Could you check a few things on this drawing? It's one solid part, dimensions in mm from its lowest x, y, z. Give positions to 0.01 mm unless a question says otherwise; leave off trailing zeros. Order: outer loops, then holes, each group sorted by start corner. A loop starts at its lowest first (then second) coordinate and runs counter-clockwise, first axis right, second up. Notation, with made-up numbers: (-19, 0) -> (9, 0) arc R19 cw to (9, 24) -> close; hole circle Ø11 at (67, 85.25). An arc over 180 degrees is marked (long way). Use one line per item in the form item = value. Start each with the question number.
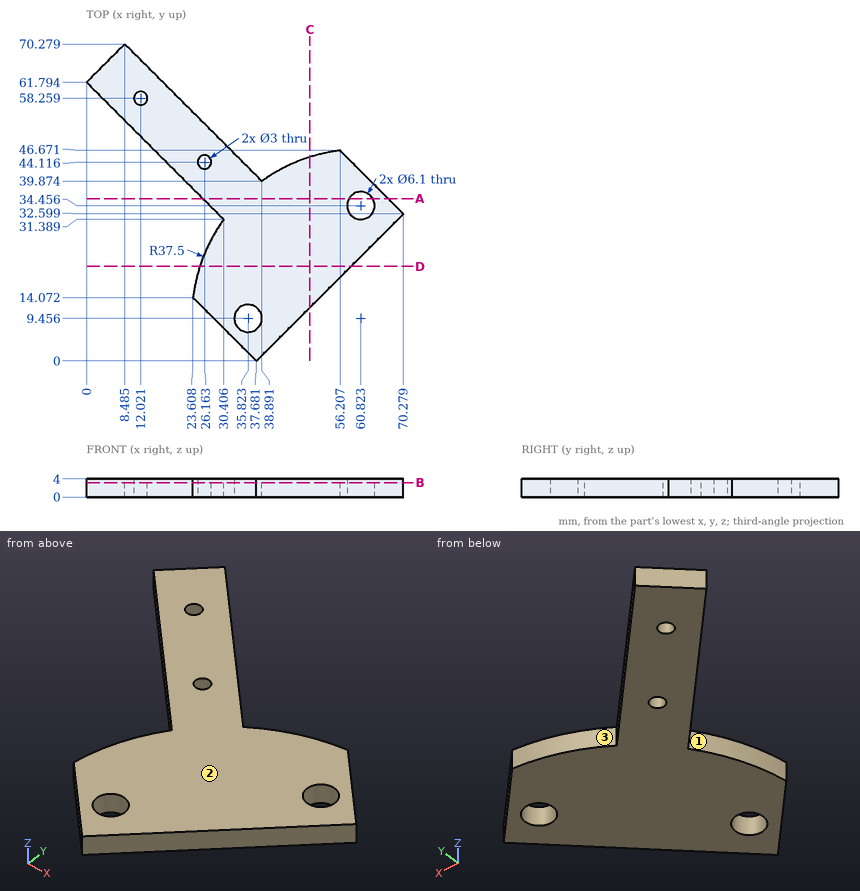
(1) I'm going to push flat-ended pins straight in: pin 1 Ø2.5 at (x, y) = (26.16, 44.12) entering from +Z; pin 2 Ø1 at (x, z) = (25, 3.5) entering from -Y; pin 3 Ø2 at (x, z) = (16.5, 3) entering from -Y (1 decimal). Where does each tip first touch, or does it pass through?
(2) Please list where these lines run through material, in increasing order: probe 1 along Y at (x, z) = (35.5, 3.35) (1 decimal); probe 2 along X at (y, z) = (40, 1.7) (1 decimal); probe 3 along X at (y, z) = (34, 1.95) (1 decimal).
(3) Imagine slicing it at D-D (y = 21). Write out the boundary of the cut face in (x, z) (1 decimal).
(4) Imagine slicing it at C-C (x = 49.5). Write out the boundary of the cut face in (y, z) (1 decimal).
(5) We'd pull the mould along X, two halves only. Please class the marked faces 1, 2 and 3: pulls with the +X half, pulls with the -X half, needs draft (parallel to the pull), parting line crosses it, or undercut.
(6) Imagine slicing it at A-A (y = 36). Write out the boundary of the cut face in (x, z) (1 decimal).
(7) Imagine slicing it at B-B (z = 3.2). Give the number of separate pieces and of enclosed holes in the cut face, plus the area to 3 significant figures.
Calculated:
q1.pin_1 = through
q1.pin_2 = 12.18
q1.pin_3 = 44.3
q2.probe_1 = 2.2 to 6.4, 12.5 to 43.3
q2.probe_2 = 21.8 to 38.8, 39.1 to 62.9
q2.probe_3 = 27.8 to 57.8, 63.8 to 68.9
q3.outline = (25.1, 0) -> (58.7, 0) -> (58.7, 4) -> (25.1, 4) -> close
q4.outline = (11.8, 0) -> (45.2, 0) -> (45.2, 4) -> (11.8, 4) -> close
q5.face_1 = pulls with the -X half
q5.face_2 = needs draft
q5.face_3 = undercut
q6.outline = (25.8, 0) -> (58.2, 0) -> (58.2, 4) -> (25.8, 4) -> close; (63.5, 0) -> (66.9, 0) -> (66.9, 4) -> (63.5, 4) -> close
q7.separate_pieces = 1
q7.enclosed_holes = 4
q7.area = 1,610 mm2
